CAD build for the part. Positions are in the model's coordinates, mm. Face numbers are marked on the shaded views. A direction names the side the tool comes from. Round coordinates to 2 decimals unless told otherwise and drop trailing zeros. Loops run counter-clockwise (first coordinate to the right, second up) from the corner with the lowest first, then second, coordinate; pieces in that order, holes last.
from build123d import *

# Parameters (mm, degrees)
F0_W     = 63.5
F0_H     = 63.5
F1_DEPTH = 1.524
F2_W     = 63.5
F2_H     = 63.5
F2_W_2   = 60.452
F2_H_2   = 60.452
F3_DEPTH = 25.4
F4_R     = 2.54
F5_R     = 1.27


with BuildPart() as f1:
    # F0 (on Top) → F1 (new body)
    with BuildSketch(Plane.XY):
        Rectangle(F0_W, F0_H)
    extrude(amount=F1_DEPTH)

    # F2 (on face) → F3 (join)
    with BuildSketch(Plane.XY.offset(1.524)):
        Rectangle(F2_W, F2_H)
        Rectangle(F2_W_2, F2_H_2, mode=Mode.SUBTRACT)
    extrude(amount=F3_DEPTH)

    # F4
    f4_edges = [f1.edges().sort_by_distance(p)[0] for p in [
        (0, 30.226, 1.524),
        (30.226, 0, 1.524),
        (0, -30.226, 1.524),
        (-30.226, 0, 1.524),
        (-30.226, 30.226, 14.224),
        (30.226, 30.226, 14.224),
        (30.226, -30.226, 14.224),
        (-30.226, -30.226, 14.224),
    ]]
    fillet(f4_edges, radius=F4_R)

    # F5
    f5_edges = [f1.edges().sort_by_distance(p)[0] for p in [
        (-30.226, 0, 26.924),
    ]]
    fillet(f5_edges, radius=F5_R)


solid = f1.part
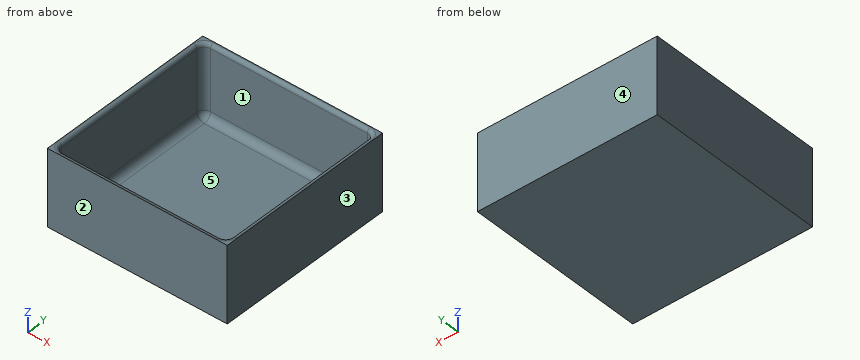
Item 1: Cut at B-B (x = -1.5). List the corners of the cut face in (y, z).
Verdict:
outline: (-31.75, 0) - (31.75, 0) - (31.75, 26.92) - (31.5, 26.92) arc R1.27 ccw to (30.23, 25.65) - (30.23, 4.06) arc R2.54 cw to (27.69, 1.52) - (-27.69, 1.52) arc R2.54 cw to (-30.23, 4.06) - (-30.23, 25.65) arc R1.27 ccw to (-31.5, 26.92) - (-31.75, 26.92) - close
Item 2: 3-axis set-ups, long thin cutter, end or side, ignore diameter. For the marked faces 4 and 5: which of +Z, -Z, +X, -X, +Y, -Y reach the whole face in a straight line?
Verdict:
face 4: +Z, -Z, +X, -X, +Y
face 5: +Z
Item 3: Flat gauge pin, fed straight in: P1, Ø6, axis at x = 16.5, y = -14, coming from the +Z side. Where does the tip first touch, or does it go through?
Verdict:
P1: stops at z = 1.52
Item 4: Wall check: L1, parallel to X at y = -20, z = 21.5; L2, parallel to Z at x = 3, y = 28. Give the ranges that are in metal, low to high.
Verdict:
L1: x = -31.75 to -30.23, 30.23 to 31.75
L2: z = 0 to 1.54
Item 5: Mould opens along Y. For the marked faces 1, 2 and 3 say: released by +Y, released by -Y, zero draft, split by the parting line, or undercut.
Verdict:
face 1: undercut
face 2: released by -Y
face 3: zero draft
Item 6: Cut at A-A (z = 10.5). List the corners of the cut face in (x, y), plus the area to 3 significant figures.
Verdict:
outline: (-31.75, -31.75) - (31.75, -31.75) - (31.75, 31.75) - (-31.75, 31.75) - close; hole (-30.23, -27.69) arc R2.54 ccw to (-27.69, -30.23) - (27.69, -30.23) arc R2.54 ccw to (30.23, -27.69) - (30.23, 27.69) arc R2.54 ccw to (27.69, 30.23) - (-27.69, 30.23) arc R2.54 ccw to (-30.23, 27.69) - close
area: 383 mm2
